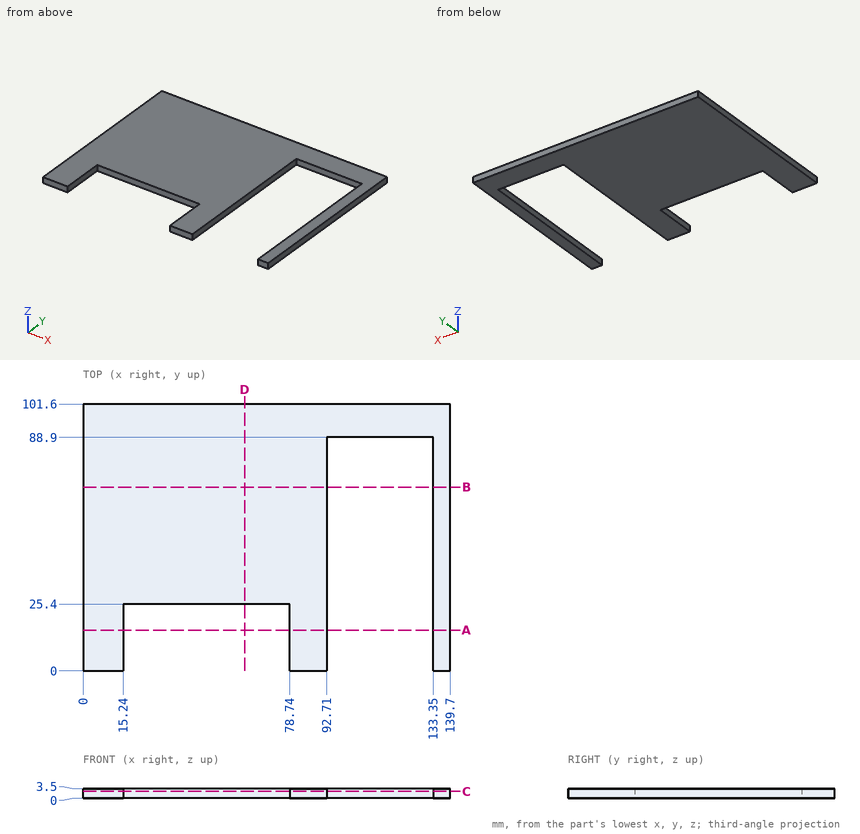
Geometry check sheet. Reference: drawing and pictorial views, mm from the part's lowest x, y, z. Coordinates: 2 decimals unless noted, no trailing zeros. Order: outer loops, then holes, each group sorted by start corner. A loop starts at its lowest first (then second) coordinate and runs counter-clockwise, first axis right, second up.
Item 1: Section check D-D (x = 61.5). Enter the section's corners in (y, z).
Item 2: Section check A-A (y = 15.5). Enter the section's corners in (x, z).
Item 3: Scan lines: line 1 along X through (y, z) = (10, 1.95); line 2 along X through (y, z) = (39, 0.8); line 3 along Y through (x, z) = (64.5, 0.85). Record each from-to range of solid material in increasing order.
Item 4: Section check C-C (z = 2.55). Enter the section's corners in (x, y).
Item 5: Section check B-B (y = 70). Enter the section's corners in (x, z), plus the area to 3 significant figures.
Item 6: Depth check by flat-ended pin: pin 1 (1.8 mm diameter, centred on y = 63, z = 1.5, fed in from -X). Enter the tip coordinate at first touch or a pass-through.
Check sheet entries:
1. outline: (25.4, 0) - (101.6, 0) - (101.6, 3.5) - (25.4, 3.5) - close
2. outline: (0, 0) - (15.24, 0) - (15.24, 3.5) - (0, 3.5) - close; (78.74, 0) - (92.71, 0) - (92.71, 3.5) - (78.74, 3.5) - close; (133.35, 0) - (139.7, 0) - (139.7, 3.5) - (133.35, 3.5) - close
3. line 1: x = 0 to 15.24, 78.74 to 92.71, 133.35 to 139.7
3. line 2: x = 0 to 92.71, 133.35 to 139.7
3. line 3: y = 25.4 to 101.6
4. outline: (0, 0) - (15.24, 0) - (15.24, 25.4) - (78.74, 25.4) - (78.74, 0) - (92.71, 0) - (92.71, 88.9) - (133.35, 88.9) - (133.35, 0) - (139.7, 0) - (139.7, 101.6) - (0, 101.6) - close
5. outline: (0, 0) - (92.71, 0) - (92.71, 3.5) - (0, 3.5) - close; (133.35, 0) - (139.7, 0) - (139.7, 3.5) - (133.35, 3.5) - close
5. area: 347 mm2
6. pin 1: stops at x = 0
